For this review, take the finished solid that the model builds, in its own axes (mm). Face numbers are marked on the shaded views. A direction names the side the tool comes from. Coordinates: 2 decimals unless noted, no trailing zeros. Loops run counter-clockwise (first coordinate to the right, second up) from the corner with the lowest first, then second, coordinate; pieces in that order, holes last. Notation, with made-up numbers: (-6, -26.75) - (32, -26.75) arc R22 cw to (32, 2.25) - close; hole circle Ø11 at (69.25, 53). An arc over 180 degrees is marked (long way). Answer as a JSON object with one key per item and string values. Group by question number.
Item 1: We need section A-A (x = 0). Give the boundary of the cut face in (y, z), then the cut area to 3 significant figures.
Item 2: To check wall thickness, follow line 1 (Y direction, x = 0, z = 23); line 2 (Y direction, x = -1, z = 28.5); line 3 (Z direction, x = 3, y = 18.5). State the ranges of each line that lie inside material, in increasing order.
Item 3: Tool access review of the marked faces 1 and 2: name each direction out of +Z, -Z, +X, -X, +Y, -Y from which nothing blocks a thin tool from reaching the whole face with its end or side.
Item 4: Mouldability with a two-part tool opening along X and no side actions: class the marked faces 3, 4 and 5 as released by +X, released by -X, zero draft, split by the parting line, or undercut.
Item 5: Clearance check with flat-ended pins moving along their axes: pin 1 (3 mm diameter, centred on x = -10, z = 21.5, fed in from -Y); pin 2 (12 mm diameter, centred on y = 2.5, z = 14, fed in from +X); pin 3 (15 mm diameter, centred on x = 11.5, y = -7, fed in from -Z). State where each tip first meets the part, or that it passes through.
Item 6: We need section D-D (x = -30). Give the boundary of the cut face in (y, z), then the cut area to 3 significant figures.
Item 7: We need section B-B (z = 18). Give the boundary of the cut face in (x, y), then the cut area to 3 significant figures.
from build123d import *

# Parameters (mm, degrees)
F0_R     = 43.410456
F1_DEPTH = 2.286
F2_R     = 33.613067
F3_DEPTH = 64.516
F4_R     = 24.771227
F5_DEPTH = 55.88


with BuildPart() as f1:
    # F0 (on Top) → F1 (new body)
    with BuildSketch(Plane.XY):
        Circle(F0_R)
    extrude(amount=F1_DEPTH)

    # F2 (on face) → F3 (join)
    with BuildSketch(Plane.XY.offset(2.286)):
        Circle(F2_R)
    extrude(amount=F3_DEPTH)

    # F4 (on Top) → F5 (cut)
    with BuildSketch(Plane.XY):
        Circle(F4_R)
    extrude(amount=F5_DEPTH, mode=Mode.SUBTRACT)


solid = f1.part
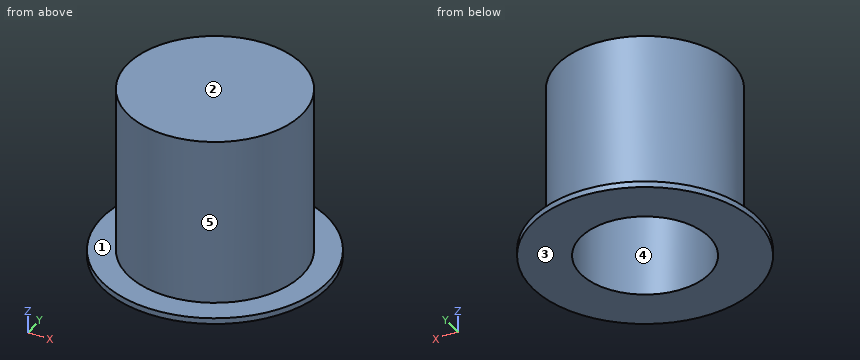
Check sheet entries:
{
 "1": {"outline": "(-43.41, 0) - (-24.77, 0) - (-24.77, 55.88) - (24.77, 55.88) - (24.77, 0) - (43.41, 0) - (43.41, 2.29) - (33.61, 2.29) - (33.61, 66.8) - (-33.61, 66.8) - (-33.61, 2.29) - (-43.41, 2.29) - close", "area": "1,770 mm2"},
 "2": {"line 1": "y = -33.61 to -24.77, 24.77 to 33.61", "line 2": "y = -33.6 to -24.75, 24.75 to 33.6", "line 3": "z = 55.88 to 66.8"},
 "3": {"face 1": "+Z", "face 2": "+Z, +X, -X, +Y, -Y"},
 "4": {"face 3": "zero draft", "face 4": "undercut", "face 5": "split by the parting line"},
 "5": {"pin 1": "stops at y = -32.52", "pin 2": "stops at x = 33.61", "pin 3": "stops at z = 55.88"},
 "6": {"outline": "(-31.38, 0) - (31.38, 0) - (31.38, 2.29) - (15.16, 2.29) - (15.16, 66.8) - (-15.16, 66.8) - (-15.16, 2.29) - (-31.38, 2.29) - close", "area": "2,100 mm2"},
 "7": {"outline": "circle Ø67.23 at (0, 0); hole circle Ø49.54 at (0, 0)", "area": "1,620 mm2"}
}
